The drawing under review shows one solid part. Ordinate dimensions are in mm from its lowest x, y, z. A direction names the side the tool comes from. Give positions to 0.01 mm unless a question says otherwise; leave off trailing zeros. Order: outer loops, then holes, each group sorted by start corner. A loop starts at its lowest first (then second) coordinate and runs counter-clockwise, first axis right, second up. Notation, with made-up numbers: (44.5, 58) -> (74.5, 58) arc R17 ccw to (74.5, 82) -> close; hole circle Ø10 at (55, 21). An arc over 180 degrees is marked (long way). Use a Markdown table: item, result. Add a question column.
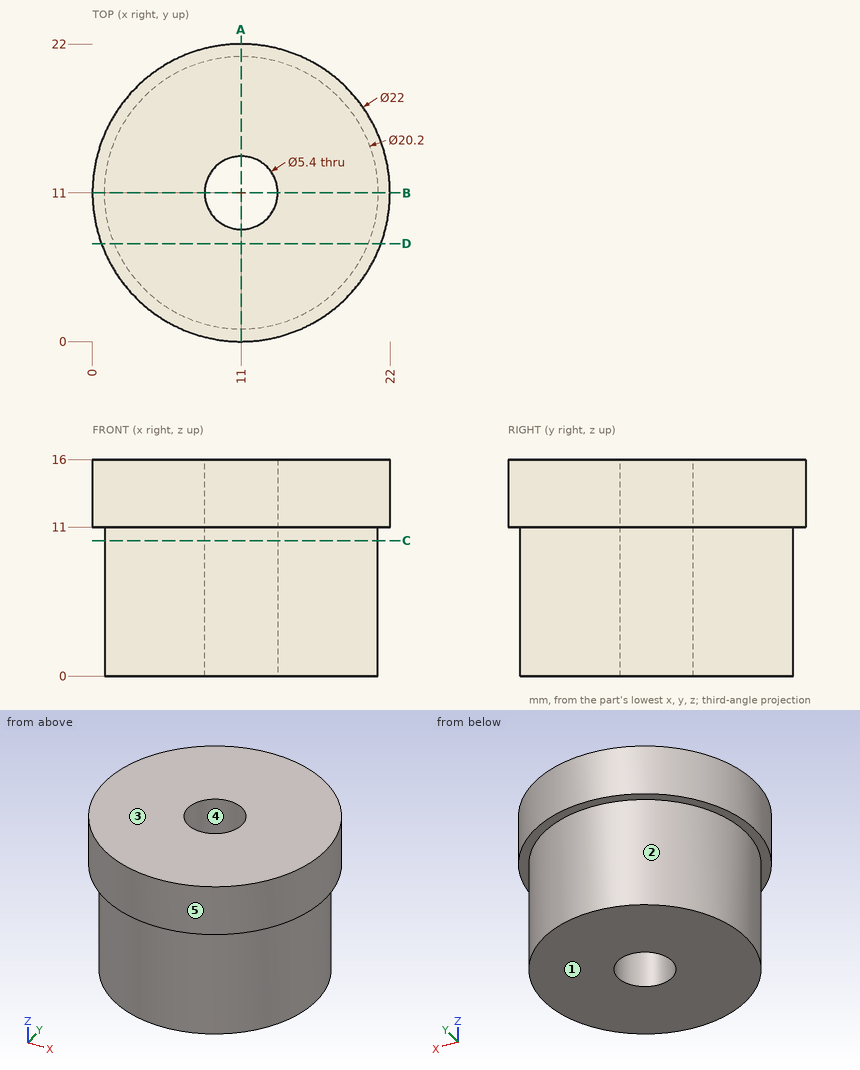
1) Add section D-D (y = 7.25). Give the boundary of the cut face in (x, z), then the cut area to 3 significant figures.
2) For L1, parallel to Y at x = 11, z = 4.75; L2, parallel to Y at x = 11, z = 11.5; L3, parallel to Z at x = 16, y = 20.25, list the stretches that pass through material, from the lowest coordinate up. Write a range as [from, to].
3) Add section A-A (x = 11). Give the boundary of the cut face in (y, z).
4) The part is to be moulded in two halves that separate along Y. For the marked faces 3, 4 and 5, say which applies: +Y half, -Y half, draft (parallel to the pull), parting line (faces both ways), or undercut.
5) Insertion check: pin 1 (3 mm diameter, centred on y = 16, z = 8, fed in from -X); pin 2 (4 mm diameter, centred on y = 6.5, z = 7, fed in from -X); pin 3 (5 mm diameter, centred on y = 4, z = 8.5, fed in from +X). Each pin has a flat end and moves straight along its axis. Give the tip position at first contact, or say it passes through.
6) Add section C-C (z = 10). Give the boundary of the cut face in (x, y), then the cut area to 3 significant figures.
7) Machinability: for the marked faces 1 and 2, which of the approach directions +Z, -Z, +X, -X, +Y, -Y give a long, thin tool a straight path to every point of the face, cutting with its end or side? Answer none if there is none.
Worked answers:
| question | item | result |
|---|---|---|
| 1 | outline | (0.66, 11) -> (1.62, 11) -> (1.62, 0) -> (20.38, 0) -> (20.38, 11) -> (21.34, 11) -> (21.34, 16) -> (0.66, 16) -> close |
| 1 | area | 310 mm^2 |
| 2 | L1 | [0.9, 8.3], [13.7, 21.1] |
| 2 | L2 | [0, 8.3], [13.7, 22] |
| 2 | L3 | [11, 16] |
| 3 | outline | (0, 11) -> (0.9, 11) -> (0.9, 0) -> (8.3, 0) -> (8.3, 16) -> (0, 16) -> close; (13.7, 0) -> (21.1, 0) -> (21.1, 11) -> (22, 11) -> (22, 16) -> (13.7, 16) -> close |
| 4 | face 3 | draft |
| 4 | face 4 | undercut |
| 4 | face 5 | parting line |
| 5 | pin 1 | x = 1.53 |
| 5 | pin 2 | x = 1.21 |
| 5 | pin 3 | x = 20.04 |
| 6 | outline | circle Ø20.2 at (11, 11); hole circle Ø5.4 at (11, 11) |
| 6 | area | 298 mm^2 |
| 7 | face 1 | -Z, +X, -X, +Y, -Y |
| 7 | face 2 | -Z |
